CAD build for the part. Positions are in the model's coordinates, mm. Face numbers are marked on the shaded views. A direction names the side the tool comes from. Give positions to 0.01 mm unless a question says otherwise; leave off trailing zeros. Loops run counter-clockwise (first coordinate to the right, second up) from the corner with the lowest first, then second, coordinate; pieces in that order, holes last. Notation, with made-up numbers: M 69,39.25 L 83,39.25 A21 ccw 83,57.25 Z; hole C 23.25,5.5 d4. An arc over 180 degrees is marked long. Answer as CSV lines item,"result".
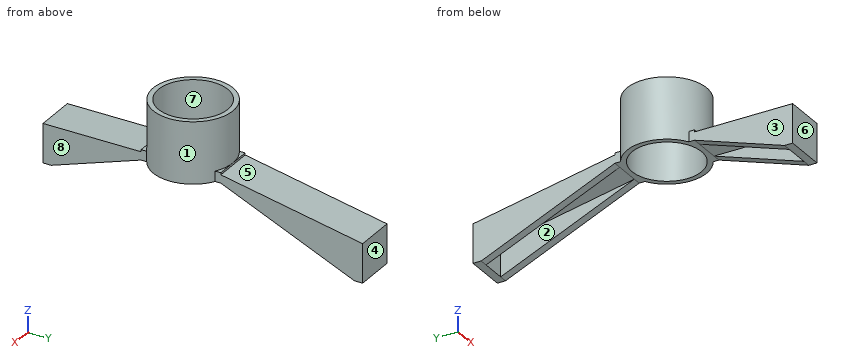
```python
from build123d import *

# Parameters (mm, degrees)
SKETCH2_R           = 39
SKETCH2_R_2         = 34
BOSS_EXTRUDE1_DEPTH = 60
BOSS_EXTRUDE2_DEPTH = 20
BOSS_EXTRUDE3_DEPTH = 10
BOSS_EXTRUDE4_DEPTH = 20
BOSS_EXTRUDE5_DEPTH = 10
BOSS_EXTRUDE6_DEPTH = 8
BOSS_EXTRUDE7_DEPTH = 8
BOSS_EXTRUDE8_DEPTH = 8
BOSS_EXTRUDE9_DEPTH = 8


with BuildPart() as part:
    # Sketch2 → Boss-Extrude1 (new body)
    with BuildSketch(Plane.XY):
        Circle(SKETCH2_R)
        Circle(SKETCH2_R_2, mode=Mode.SUBTRACT)
    extrude(amount=BOSS_EXTRUDE1_DEPTH)



with BuildPart() as body_2:
    # Sketch4 → Boss-Extrude2 (new, symmetric)
    with BuildSketch(Plane(origin=(0, 0, 0), x_dir=(0, 0, -1), z_dir=(1, 0, 0))):
        Polygon((-8, 39), (18.753791407, 177.8), (56.753791407, 177.8), (56.753791407, 169.8), (25.211786138, 169.8), (0, 39), align=None)
    extrude(amount=BOSS_EXTRUDE2_DEPTH, both=True)


with BuildPart() as part_1:
    add(part.part)

    add(body_2.part)  # Boss-Extrude3 merges body 2
    # Sketch5 → Boss-Extrude3 (add)
    with BuildSketch(Plane(origin=(0, 0, 0), x_dir=(-1, 0, 0), z_dir=(0, 0, -1))):
        with BuildLine():
            Line((0, 39), (-20, 39))
            Line((-20, 39), (-20, 33.481338086))
            ThreePointArc((-20, 33.481338086), (-10.373712322, 37.595027499), (0, 39))
        make_face()
        with BuildLine():
            Line((20, 39), (0, 39))
            ThreePointArc((0, 39), (10.373712322, 37.595027499), (20, 33.481338086))
            Line((20, 33.481338086), (20, 39))
        make_face()
    extrude(amount=-BOSS_EXTRUDE3_DEPTH)



with BuildPart() as body_2_2:
    # Sketch7 → Boss-Extrude4 (new, symmetric)
    with BuildSketch(Plane(origin=(0, 0, 0), x_dir=(0, 0, -1), z_dir=(1, 0, 0))):
        Polygon((-8, -39), (-7.916224207, -134.999963446), (30.083775793, -134.999963446), (30.092153418, -127), (0.092153418, -127), (0, -39), align=None)
    extrude(amount=BOSS_EXTRUDE4_DEPTH, both=True)


with BuildPart() as part_2:
    add(part_1.part)

    add(body_2_2.part)  # Boss-Extrude5 merges body 2 2
    # Sketch8 → Boss-Extrude5 (add)
    with BuildSketch(Plane(origin=(0, 0, 0), x_dir=(-1, 0, 0), z_dir=(0, 0, -1))):
        with BuildLine():
            Line((-20, -33.481338086), (-20, -39))
            Line((-20, -39), (0, -39))
            ThreePointArc((0, -39), (-10.373712322, -37.595027499), (-20, -33.481338086))
        make_face()
        with BuildLine():
            ThreePointArc((20, -33.481338086), (10.373712322, -37.595027499), (0, -39))
            Line((0, -39), (20, -39))
            Line((20, -39), (20, -33.481338086))
        make_face()
    extrude(amount=-BOSS_EXTRUDE5_DEPTH)

    # Sketch9 → Boss-Extrude6 (add)
    with BuildSketch(Plane(origin=(20, 0, 0), x_dir=(0, 0, -1), z_dir=(1, 0, 0))):
        Polygon((56.753791407, 169.8), (0, 39), (25.211786138, 169.8), align=None)
    extrude(amount=-BOSS_EXTRUDE6_DEPTH)

    # Sketch10 → Boss-Extrude7 (add)
    with BuildSketch(Plane.ZY.offset(20)):
        Polygon((0, 39), (-25.211786138, 169.8), (-56.753791407, 169.8), align=None)
    extrude(amount=-BOSS_EXTRUDE7_DEPTH)

    # Sketch11 → Boss-Extrude8 (add)
    with BuildSketch(Plane(origin=(20, 0, 0), x_dir=(0, 0, -1), z_dir=(1, 0, 0))):
        Polygon((0, -39), (30.092153418, -127), (0.092153418, -127), align=None)
    extrude(amount=-BOSS_EXTRUDE8_DEPTH)

    # Sketch12 → Boss-Extrude9 (add)
    with BuildSketch(Plane.ZY.offset(20)):
        Polygon((-30.092153418, -127), (-0.092153418, -127), (0, -39), align=None)
    extrude(amount=-BOSS_EXTRUDE9_DEPTH)


solid = part_2.part
```
Q1. Mould opens along Y. For the marked faces 6, 7 and 8 say: released by +Y, released by -Y, zero draft, split by the parting line, or undercut.
Solution:
face 6,"released by -Y"
face 7,"undercut"
face 8,"zero draft"
Q2. Cut at B-B (x = -30.5). Write the cut outline in (y, z), and give its area (3 significant figures).
Solution:
outline,"M -24.31,0 L -15.02,0 L -15.02,60 L -24.31,60 Z; M 15.02,0 L 24.31,0 L 24.31,60 L 15.02,60 Z"
area,"1,110 mm²"
Q3. Cut at C-C (z = 53.5). Write the cut outline in (x, y), and give its area (3 significant figures).
Solution:
outline,"C 0,0 d78; hole C 0,0 d68"
area,"1,150 mm²"
Q4. Wall check: line 1 (Y direction, x = 0, z = 25.5); line 2 (X direction, y = -77.5, z = -9.5); line 3 (Y direction, x = 23.5, z = 36). Give the ranges that are in metal, low to high. Write a range as [from, to].
Solution:
line 1,"y = [-39, -34], [34, 39]"
line 2,"x = [-20, -12], [12, 20]"
line 3,"y = [-31.12, -24.57], [24.57, 31.12]"
Q5. Cut at D-D (z = -37). Write the cut outline in (x, y).
Solution:
outline,"M -20,124.27 L -12,124.27 L -12,169.8 L 12,169.8 L 12,124.27 L 20,124.27 L 20,177.8 L -20,177.8 Z"
Q6. Cut at A-A (y = 0). Write the cut outline in (x, z), and give its area (3 significant figures).
Solution:
outline,"M -39,0 L -34,0 L -34,60 L -39,60 Z; M 34,0 L 39,0 L 39,60 L 34,60 Z"
area,"600 mm²"
Q7. Pin check, flat tips, straight feed: P1, Ø12, axis at y = -101, z = -11, coming from the -X side; P2, Ø24, axis at y = -80.5, z = -13, coming from the +X side; P3, Ø8, axis at x = 0, z = 44, coming from the +Y side. Stop position of each tip, or through.
Solution:
P1,"stops at x = -20"
P2,"stops at x = 20"
P3,"stops at y = 39"
Q8. Which spindle directions (+Z, -Z, +X, -X, +Y, -Y) get a long thin tool onto all of the face, cutting with end or side? Do the marked faces 1, 2, 3, 4 and 5. Say none if no direction does.
Solution:
face 1,"+Z"
face 2,"-Z"
face 3,"+Z, -Z, -X, -Y"
face 4,"+Z, -Z, +X, -X, +Y"
face 5,"+Z, +X, -X, +Y"
